from build123d import *

# Parameters (mm, degrees)
SKETCH_1_R          = 1.6
EXTRUDE_1_DEPTH     = 5
SKETCH_2_R          = 2.9
CUT_EXTRUDE_1_DEPTH = 2
CUT_EXTRUDE_3_DEPTH = 71.600960604
FILLET_1_R          = 5
FILLET_2_R          = 3
FILLET_4_R          = 2
FILLET_6_R          = 2
FILLET_7_R          = 2
FILLET_8_R          = 3


with BuildPart() as part:
    # 草图1 → 凸台-拉伸1 (new body)
    with BuildSketch(Plane.XY):
        with BuildLine():
            Line((-41.565100182, -49.426292213), (-39.485969284, -49.426292213))
            Line((-39.485969284, -49.426292213), (-13.65407564, -49.426292213))
            Line((-13.65407564, -49.426292213), (-11.764178943, -49.426292213))
            ThreePointArc((-11.764178943, -49.426292213), (-8.228645037, -47.961826119), (-6.764178943, -44.426292213))
            Line((-6.764178943, -44.426292213), (-6.764178943, -42.471801942))
            Line((-6.764178943, -42.471801942), (-6.761688654, -42.088770435))
            ThreePointArc((-6.761688654, -42.088770435), (-7.959392434, -38.809211433), (-11.011044569, -37.112915219))
            ThreePointArc((-11.011044569, -37.112915219), (-17.52195854, -35.410370983), (-23.534396799, -32.386921995))
            ThreePointArc((-23.534396799, -32.386921995), (-36.041802291, -31.338005667), (-35.33797784, -18.806443564))
            ThreePointArc((-35.33797784, -18.806443564), (-36.996722237, -14.362622261), (-37.982061376, -9.722785245))
            ThreePointArc((-37.982061376, -9.722785245), (-39.647864751, -6.630640555), (-42.936394307, -5.397014589))
            Line((-42.936394307, -5.397014589), (-45.165100182, -5.397014589))
            ThreePointArc((-45.165100182, -5.397014589), (-48.700634088, -6.861480683), (-50.165100182, -10.397014589))
            Line((-50.165100182, -10.397014589), (-50.165100182, -15.397014589))
            Line((-50.165100182, -15.397014589), (-50.165100182, -25.564927735))
            Line((-50.165100182, -25.564927735), (-50.165100182, -38.747161315))
            Line((-50.165100182, -38.747161315), (-50.165100182, -41.426292213))
            Line((-50.165100182, -41.426292213), (-50.165100182, -46.426292213))
            Line((-50.165100182, -46.426292213), (-45.165100182, -46.426292213))
            Line((-45.165100182, -46.426292213), (-41.565100182, -46.426292213))
            Line((-41.565100182, -46.426292213), (-41.565100182, -49.426292213))
        make_face()
        with Locations((-44.74192859, -40.941023834)):
            Circle(SKETCH_1_R, mode=Mode.SUBTRACT)
        with BuildLine():
            ThreePointArc((-27.889312547, -46.323727421), (-29.989312547, -44.223727421), (-27.889312547, -42.123727421))
            Line((-27.889312547, -42.123727421), (-22.889312547, -42.123727421))
            ThreePointArc((-22.889312547, -42.123727421), (-20.789312547, -44.223727421), (-22.889312547, -46.323727421))
            Line((-22.889312547, -46.323727421), (-27.889312547, -46.323727421))
        make_face(mode=Mode.SUBTRACT)
        with Locations((-13.741931799, -40.926918244)):
            Circle(SKETCH_1_R, mode=Mode.SUBTRACT)
        with BuildLine():
            ThreePointArc((-46.565100182, -27.664927735), (-48.665100182, -25.564927735), (-46.565100182, -23.464927735))
            Line((-46.565100182, -23.464927735), (-41.565100182, -23.464927735))
            ThreePointArc((-41.565100182, -23.464927735), (-39.465100182, -25.564927735), (-41.565100182, -27.664927735))
            Line((-41.565100182, -27.664927735), (-46.565100182, -27.664927735))
        make_face(mode=Mode.SUBTRACT)
        with Locations((-44.756034179, -9.941027044)):
            Circle(SKETCH_1_R, mode=Mode.SUBTRACT)
    extrude(amount=EXTRUDE_1_DEPTH)

    # 草图2 → 切除-拉伸1 (cut)
    with BuildSketch(Plane(origin=(0, 0, 5), x_dir=(-1, 0, 0), z_dir=(0, 0, -1))):
        with Locations((44.756034179, -9.941027044)):
            Circle(SKETCH_2_R)
        with Locations((44.74192859, -40.941023834)):
            Circle(SKETCH_2_R)
        with Locations((13.741931799, -40.926918244)):
            Circle(SKETCH_2_R)
    extrude(amount=CUT_EXTRUDE_1_DEPTH, mode=Mode.SUBTRACT)

    # 草图3 → 切除-拉伸3 (cut, through all)
    with BuildSketch(Plane(origin=(0, 0, 0), x_dir=(-1, 0, 0), z_dir=(0, 0, -1))):
        Polygon((8.241263234, -42.394978236), (12.268866598, -46.426248541), (15.268866287, -49.426292213), (33.268866287, -49.426292213), (33.268866287, -44.726292213), (48.610476999, -44.726292213), (50.241258886, -44.726292213), (50.241258886, -51.356689398), (5.002855071, -51.356689398), (5.002855071, -38.135185544), (8.243201521, -38.135185544), align=None)
    extrude(amount=-CUT_EXTRUDE_3_DEPTH, mode=Mode.SUBTRACT)

    # 圆角1
    fillet_1_edges = [part.edges().sort_by_distance(p)[0] for p in [
        (-8.241263234, -42.394978236, 2.5),
        (-15.268866287, -49.426292213, 2.5),
    ]]
    fillet(fillet_1_edges, radius=FILLET_1_R)

    # 圆角2
    fillet_2_edges = [part.edges().sort_by_distance(p)[0] for p in [
        (-8.243033782, -38.503826079, 2.5),
    ]]
    fillet(fillet_2_edges, radius=FILLET_2_R)

    # 圆角4
    fillet_4_edges = [part.edges().sort_by_distance(p)[0] for p in [
        (-33.268866287, -49.426292213, 2.5),
    ]]
    fillet(fillet_4_edges, radius=FILLET_4_R)

    # 圆角6
    fillet_6_edges = [part.edges().sort_by_distance(p)[0] for p in [
        (-33.268866287, -44.726292213, 2.5),
    ]]
    fillet(fillet_6_edges, radius=FILLET_6_R)

    # 圆角7
    fillet_7_edges = [part.edges().sort_by_distance(p)[0] for p in [
        (-23.534396799, -32.386921995, 2.5),
        (-35.33797784, -18.806443564, 2.5),
    ]]
    fillet(fillet_7_edges, radius=FILLET_7_R)

    # 圆角8
    fillet_8_edges = [part.edges().sort_by_distance(p)[0] for p in [
        (-50.165100182, -44.726292213, 2.5),
    ]]
    fillet(fillet_8_edges, radius=FILLET_8_R)


solid = part.part
Source: CAD feature listing. Evaluate the final solid. Frame: model axes, mm. A direction names the side the tool comes from. Round coordinates to 2 decimals unless told otherwise and drop trailing zeros. Loops run counter-clockwise (first coordinate to the right, second up) from the corner with the lowest first, then second, coordinate; pieces in that order, holes last. Notation, with made-up numbers: (61, 46.25) - (65, 46.25) arc R21 cw to (65, 76.25) - close; hole circle Ø10 at (-9, -12.75). An arc over 180 degrees is marked (long way). Write item = value, one per line. Start each with the question number.
(1) Section query C-C, the plane x = -27. Output: boundary loops of the cut face in (y, z), plus the area to 3 significant figures.
(2) Pull-direction query (X, two-part tool) for faces 1 (the face through (-49.31, -43.824, 2.535)), 2 (the face through (-42.605, -38.981, 4.014)), 3 (the face through (-44, -5.397, 2)); classes: +X half, -X half, draft (parallel to the pull), parting line (faces both ways), or undercut.
(3) Ray query, line 1 along Y through (x, z) = (-45, 4.6); line 2 along Y through (x, z) = (-29.5, 2.05); line 3 along X through (y, z) = (-39, 4.05). Return the intervals inside material, ascending. Write a range as from..to.
(4) Section query A-A, the plane y = -11. Output: boundary loops of the cut face in (x, z).
(5) Section query D-D, the plane z = 1.2. State how many separate pieces and enclosed holes the cut face has, plus the area to 3 significant figures.
(6) Set-up query: faces 4 (the face through (-32.667, -48.856, 2.535)), 5 (the face through (-46.094, -12.514, 4.014)), 6 (the face through (-44, -23.465, 2)). Return all of +Z, -Z, +X, -X, +Y, -Y with unobstructed straight access to the full face (end or side cutting, diameter ignored); none if empty.
(7) Pin query (flat end, axial travel): pin 1 (2.5 mm diameter, centred on x = -13.74, y = -40.93, fed in from -Z); pin 2 (1.7 mm diameter, centred on x = -14.5, y = -40.5, fed in from +Z); pin 3 (0.6 mm diameter, centred on y = -47, z = 2.5, fed in from -X); pin 4 (2.5 mm diameter, centred on x = -42.5, z = 3.5, fed in from -Y). Return the tip coordinate at first contact, or that it passes through.
(8) Section query B-B, the plane x = -40. Output: boundary loops of the cut face in (y, z), plus the area to 3 significant figures.
Conclusion:
q1.outline = (-49.43, 0) - (-46.32, 0) - (-46.32, 5) - (-49.43, 5) - close; (-42.12, 0) - (-34.15, 0) - (-34.15, 5) - (-42.12, 5) - close
q1.area = 55.4 mm2
q2.face_1 = -X half
q2.face_2 = undercut
q2.face_3 = draft
q3.line_1 = -44.73..-43.83, -38.05..-27.66, -23.46..-12.83, -7.05..-5.4
q3.line_2 = -49.43..-45.57, -42.88..-34.43
q3.line_3 = -50.17..-46.9, -42.59..-15.91, -11.57..-8.46
q4.outline = (-50.17, 0) - (-45.96, 0) - (-45.96, 3) - (-47.46, 3) - (-47.46, 5) - (-50.17, 5) - close; (-43.56, 0) - (-37.78, 0) - (-37.78, 5) - (-42.06, 5) - (-42.06, 3) - (-43.56, 3) - close
q5.separate_pieces = 1
q5.enclosed_holes = 5
q5.area = 783 mm2
q6.face_4 = +Z, -Z, -X, -Y
q6.face_5 = +Z
q6.face_6 = +Z, -Z
q7.pin_1 = through
q7.pin_2 = 3
q7.pin_3 = -33.27
q7.pin_4 = -44.73
q8.outline = (-44.73, 0) - (-26.97, 0) - (-26.97, 5) - (-44.73, 5) - close; (-24.16, 0) - (-6.35, 0) - (-6.35, 5) - (-24.16, 5) - close
q8.area = 178 mm2
